```python
from build123d import *

# Parameters (mm, degrees)
SKETCH1_R           = 10.9855
BOSS_EXTRUDE1_DEPTH = 40.767
SKETCH2_R           = 6.0071
BOSS_EXTRUDE2_DEPTH = 3.81
SKETCH3_R           = 2.9972
BOSS_EXTRUDE3_DEPTH = 2.54
SKETCH4_R           = 4.7625
BOSS_EXTRUDE4_DEPTH = 7.62
SKETCH5_R           = 1.5
CUT_EXTRUDE1_DEPTH  = 7.62
CIRPATTERN1_COUNT   = 4


with BuildPart() as part:
    # Sketch1 → Boss-Extrude1 (new, symmetric)
    with BuildSketch(Plane(origin=(0, 0, 0), x_dir=(1, 0, 0), z_dir=(0, 1, 0))):
        with Locations(Location((0, 0, 0), (0, 0, 270))):
            Circle(SKETCH1_R)
    extrude(amount=BOSS_EXTRUDE1_DEPTH, both=True)

    # Sketch2 → Boss-Extrude2 (add)
    with BuildSketch(Plane(origin=(0, 40.767, 0), x_dir=(1, 0, 0), z_dir=(0, 1, 0))):
        with Locations(Location((0, 0, 0), (0, 0, 90))):
            Circle(SKETCH2_R)
    extrude(amount=BOSS_EXTRUDE2_DEPTH)

    # Sketch3 → Boss-Extrude3 (add)
    with BuildSketch(Plane(origin=(0, 44.577, 0), x_dir=(1, 0, 0), z_dir=(0, 1, 0))):
        with Locations(Location((0, 0, 0), (0, 0, 270))):
            Circle(SKETCH3_R)
    extrude(amount=BOSS_EXTRUDE3_DEPTH)

    # Sketch4 → Boss-Extrude4 (add)
    with BuildSketch(Plane(origin=(0, 47.117, 0), x_dir=(1, 0, 0), z_dir=(0, 1, 0))):
        with Locations(Location((0, 0, 0), (0, 0, 90))):
            Circle(SKETCH4_R)
    extrude(amount=BOSS_EXTRUDE4_DEPTH)

    # Sketch5 → Cut-Extrude1 (cut)
    with BuildSketch(Plane(origin=(0, 40.767, 0), x_dir=(1, 0, 0), z_dir=(0, 1, 0))):
        with Locations(Location((0, 9.017, 0), (0, 0, 270))):
            Circle(SKETCH5_R)
    cut_extrude1 = extrude(amount=-CUT_EXTRUDE1_DEPTH, mode=Mode.SUBTRACT)

    # CirPattern1: Cut-Extrude1 ×4 about axis
    cirpattern1_axis = Axis((0, 0, 0), (0, 1, 0))
    for i in range(1, CIRPATTERN1_COUNT):
        add(cut_extrude1.rotate(cirpattern1_axis, i * 360 / CIRPATTERN1_COUNT), mode=Mode.SUBTRACT)


solid = part.part
```
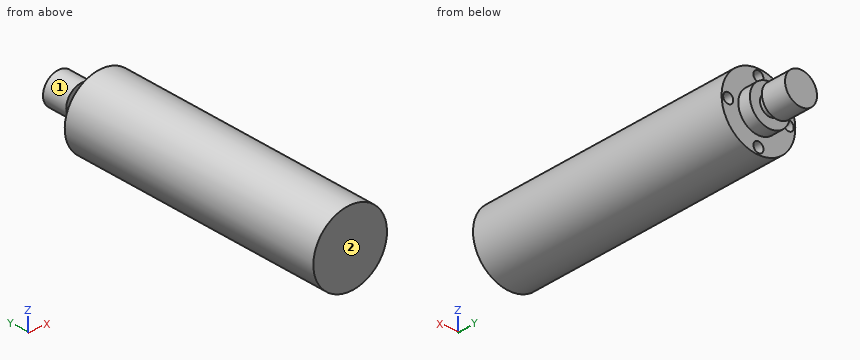
Geometry: final body of the model. Coordinates: model frame, mm. Face numbers are marked on the shaded views. A direction names the side the tool comes from. Round coordinates to 2 decimals unless told otherwise and drop trailing zeros. Order: outer loops, then holes, each group sorted by start corner. A loop starts at its lowest first (then second) coordinate and runs counter-clockwise, first axis right, second up. Notation, with made-up numbers: (-18.75, -37) -> (-14.75, -37) arc R29 ccw to (-14.75, -10) -> close; hole circle Ø9 at (-6.75, -33). An arc over 180 degrees is marked (long way). Use CSV: the item, a comma, the result in double quotes. Start each with the question number.
1) Material intervals for line 1 along Y through (x, z) = (0.75, 3); line 2 along Y through (x, z) = (9.75, 1.25); line 3 along Y through (x, z) = (-7.5, -4.5), sorted ascending. Write a range as from..to.
2) Section D-D (x = 9.25). Return the cut outline in (y, z), and give its area (3 significant figures).
3) Section C-C (y = 12). Return the cut outline in (x, z), and give its area (3 significant figures).
4) First-contact query: pin 1 Ø8 at (y, z) = (-30.5, -5) entering from +X; pin 2 Ø2.5 at (x, z) = (-0.5, -9) entering from +Y; pin 3 Ø1 at (y, z) = (21.5, -2.5) entering from -X. Flat tips, straight axial feed; report the tip coordinate or a pass-through.
5) Section A-A (x = 0). Return the cut outline in (y, z).
6) Section B-B (z = 0). Return the cut outline in (x, y).
7) Set-up query: the marked faces 1 and 2. Return all of +Z, -Z, +X, -X, +Y, -Y with unobstructed straight access to the full face (end or side cutting, diameter ignored); none if empty.
Returned:
1,line 1,"y = -40.77..44.58, 47.12..54.74"
1,line 2,"y = -40.77..33.15"
1,line 3,"y = -40.77..40.77"
2,outline,"(-40.77, -5.93) -> (40.77, -5.93) -> (40.77, -1.48) -> (33.15, -1.48) -> (33.15, 1.48) -> (40.77, 1.48) -> (40.77, 5.93) -> (-40.77, 5.93) -> close"
2,area,"944 mm²"
3,outline,"circle Ø21.97 at (0, 0)"
3,area,"379 mm²"
4,pin 1,"stops at x = 10.94"
4,pin 2,"stops at y = 40.77"
4,pin 3,"stops at x = -10.8"
5,outline,"(-40.77, -10.99) -> (40.77, -10.99) -> (40.77, -10.52) -> (33.15, -10.52) -> (33.15, -7.52) -> (40.77, -7.52) -> (40.77, -6.01) -> (44.58, -6.01) -> (44.58, -3) -> (47.12, -3) -> (47.12, -4.76) -> (54.74, -4.76) -> (54.74, 4.76) -> (47.12, 4.76) -> (47.12, 3) -> (44.58, 3) -> (44.58, 6.01) -> (40.77, 6.01) -> (40.77, 7.52) -> (33.15, 7.52) -> (33.15, 10.52) -> (40.77, 10.52) -> (40.77, 10.99) -> (-40.77, 10.99) -> close"
6,outline,"(-10.99, -40.77) -> (10.99, -40.77) -> (10.99, 40.77) -> (10.52, 40.77) -> (10.52, 33.15) -> (7.52, 33.15) -> (7.52, 40.77) -> (6.01, 40.77) -> (6.01, 44.58) -> (3, 44.58) -> (3, 47.12) -> (4.76, 47.12) -> (4.76, 54.74) -> (-4.76, 54.74) -> (-4.76, 47.12) -> (-3, 47.12) -> (-3, 44.58) -> (-6.01, 44.58) -> (-6.01, 40.77) -> (-7.52, 40.77) -> (-7.52, 33.15) -> (-10.52, 33.15) -> (-10.52, 40.77) -> (-10.99, 40.77) -> close"
7,face 1,"+Y"
7,face 2,"+Z, -Z, +X, -X, -Y"
